from build123d import *

# Parameters (mm, degrees)
F0_W     = 40.593308
F0_H     = 18.237574
F1_DEPTH = 8
F2_W     = 39.236986
F2_H     = 14.72901
F3_DEPTH = 6


with BuildPart() as f1:
    # F0 (on Top) → F1 (new body)
    with BuildSketch(Plane.XY):
        Rectangle(F0_W, F0_H)
        with BuildLine():
            Line((20.296654, 9.118787), (20.296654, -9.118787))
            ThreePointArc((20.296654, -9.118787), (29.415441, 0), (20.296654, 9.118787))
        make_face()
        with BuildLine():
            ThreePointArc((-20.296654, 9.118787), (-29.415441, 0), (-20.296654, -9.118787))
            Line((-20.296654, -9.118787), (-20.296654, 9.118787))
        make_face()
    extrude(amount=F1_DEPTH)

    # F2 (on face) → F3 (cut)
    with BuildSketch(Plane.XY.offset(8)):
        Rectangle(F2_W, F2_H)
        with BuildLine():
            Line((19.618493, 7.364505), (19.618493, -7.364505))
            ThreePointArc((19.618493, -7.364505), (26.982998, 0), (19.618493, 7.364505))
        make_face()
        with BuildLine():
            ThreePointArc((-19.618493, 7.364505), (-26.982998, 0), (-19.618493, -7.364505))
            Line((-19.618493, -7.364505), (-19.618493, 7.364505))
        make_face()
    extrude(amount=-F3_DEPTH, mode=Mode.SUBTRACT)


solid = f1.part
Verification items for the finished model (mm, model axes). A direction names the side the tool comes from. Give positions to 0.01 mm unless a question says otherwise; leave off trailing zeros. Write each loop counter-clockwise with the first axis right and the second up, starting at its lowest first coordinate (ties: lowest second). Pieces come first, ordered by that corner, then holes.
(1) Mould release check, pull along Y, two halves, no side actions. Record for faces 1 (the face through (0, 7.365, 5)), 2 (the face through (-29.413, 0.201, 3.944)), 3 (the face through (0, -9.119, 4)): +Y half, -Y half, draft (parallel to the pull), parting line (faces both ways), or undercut.
(2) Material ranges on line 1 (Y direction, x = -1, z = 6.75); line 2 (Z direction, x = 15, y = -3.5); line 3 (X direction, y = 3.5, z = 6.5), recorded low to high.
(3) Access from +Z, -Z, +X, -X, +Y, -Y to the whole of each face (thin tool, end or side, straight path). Record for faces 4 (the face through (26.98, -0.16, 5.04)), 5 (the face through (0, 0, 0)).
(4) Gauge pin test, flat ends, axial feed: pin 1 (8 mm diameter, centred on x = -4.5, y = -3, fed in from -Z); pin 2 (2 mm diameter, centred on y = 5.5, z = 7, fed in from +X); pin 3 (4 mm diameter, centred on y = -6.5, z = 7, fed in from -X). Record the tip position at first contact, or that the pin passes through.
(5) Cross-section at C-C (y = 0). Enter the section's corners in (x, z).
(6) Cross-section at A-A (x = 6). Enter the section's corners in (y, z), plus the area to 3 significant figures.
(7) Cross-section at B-B (z = 5.25). Enter the section's corners in (x, y).
Worked out:
1. face 1: undercut
1. face 2: parting line
1. face 3: -Y half
2. line 1: y = -9.12 to -7.36, 7.36 to 9.12
2. line 2: z = 0 to 2
2. line 3: x = -28.72 to -26.1, 26.1 to 28.72
3. face 4: +Z
3. face 5: -Z, +X, -X, +Y, -Y
4. pin 1: stops at z = 0
4. pin 2: stops at x = 28.23
4. pin 3: stops at x = -28.23
5. outline: (-29.42, 0) - (29.42, 0) - (29.42, 8) - (26.98, 8) - (26.98, 2) - (-26.98, 2) - (-26.98, 8) - (-29.42, 8) - close
6. outline: (-9.12, 0) - (9.12, 0) - (9.12, 8) - (7.36, 8) - (7.36, 2) - (-7.36, 2) - (-7.36, 8) - (-9.12, 8) - close
6. area: 57.5 mm2
7. outline: (-20.3, -9.12) - (20.3, -9.12) arc R9.12 ccw to (20.3, 9.12) - (-20.3, 9.12) arc R9.12 ccw to start; hole (-19.62, -7.36) - (19.62, -7.36) arc R7.36 ccw to (19.62, 7.36) - (-19.62, 7.36) arc R7.36 ccw to start
